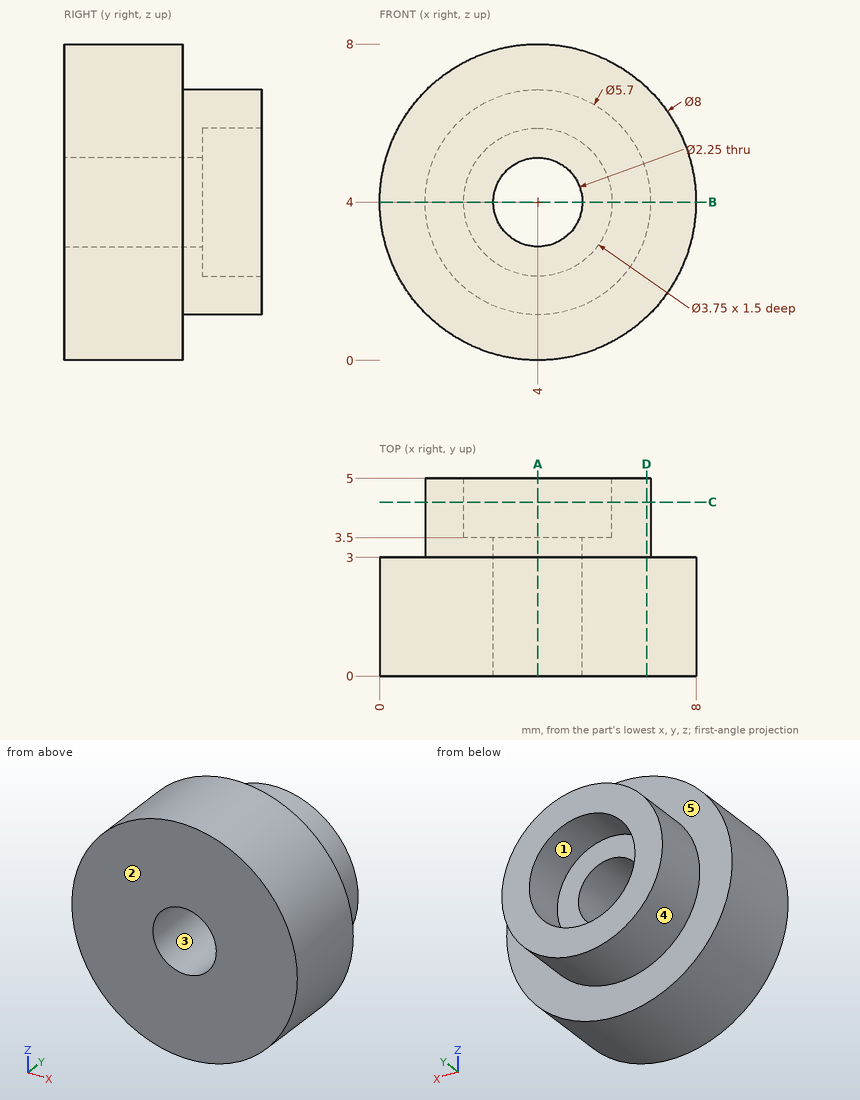
The drawing under review shows one solid part. Ordinate dimensions are in mm from its lowest x, y, z. A direction names the side the tool comes from. Round coordinates to 2 decimals unless told otherwise and drop trailing zeros. Loops run counter-clockwise (first coordinate to the right, second up) from the corner with the lowest first, then second, coordinate; pieces in that order, holes last. Notation, with made-up numbers: (23, 3) -> (66, 3) arc R29 cw to (66, 34) -> close; hole circle Ø10 at (-34, 34.25). An arc over 180 degrees is marked (long way). One line per question, with ' | ' between items. Start each with the question number.
Item 1: Add section C-C, the plane y = 4.4. Write out the cut boundary in (x, z) (3 decimals).
Item 2: Draft analysis for pull direction X (two halves, no side actions). For the marked faces 3, 4 and 5, state which applies: +X half, -X half, draft (parallel to the pull), parting line (faces both ways), or undercut.
Item 3: Add section B-B, the plane z = 4. Write out the cut boundary in (x, y) (3 decimals).
Item 4: For pin 1 (1.5 mm diameter, centred on y = 4, z = 5.5, fed in from -X); pin 2 (1.9 mm diameter, centred on x = 3.5, z = 3.5, fed in from +Y), all flat-tipped, find the tip position at first contact; note any pin that passes through.
Item 5: Add section D-D, the plane x = 6.75. Write out the cut boundary in (y, z).
Item 6: Wall thickness on line 1 along X through (y, z) = (4.1, 4) (3 decimals); line 2 along X through (y, z) = (1.15, 4) (3 decimals); line 3 along Y through (x, z) = (7, 2.5): over which ranges is each line inside the solid? List them lowest first. Write a range as [from, to].
Item 7: Machinability: for the marked faces 1 and 2, which of the approach directions +Z, -Z, +X, -X, +Y, -Y give a long, thin tool a straight path to every point of the face, cutting with its end or side? Answer none if there is none.
Item 8: Add section A-A, the plane x = 4. Write out the cut boundary in (y, z) (3 decimals), then the cut area to 3 significant figures.
Return value:
1) outline: circle Ø5.7 at (4, 4); hole circle Ø3.75 at (4, 4)
2) face 3: undercut | face 4: parting line | face 5: draft
3) outline: (0, 0) -> (2.875, 0) -> (2.875, 3.5) -> (2.125, 3.5) -> (2.125, 5) -> (1.15, 5) -> (1.15, 3) -> (0, 3) -> close; (5.125, 0) -> (8, 0) -> (8, 3) -> (6.85, 3) -> (6.85, 5) -> (5.875, 5) -> (5.875, 3.5) -> (5.125, 3.5) -> close
4) pin 1: stops at x = 1.25 | pin 2: stops at y = 3.5
5) outline: (0, 1.1) -> (3, 1.1) -> (3, 3.25) -> (5, 3.25) -> (5, 4.75) -> (3, 4.75) -> (3, 6.9) -> (0, 6.9) -> close
6) line 1: x = [1.15, 2.125], [5.875, 6.85] | line 2: x = [0, 2.875], [5.125, 8] | line 3: y = [0, 3]
7) face 1: +Y | face 2: +Z, -Z, +X, -X, -Y
8) outline: (0, 0) -> (3, 0) -> (3, 1.15) -> (5, 1.15) -> (5, 2.125) -> (3.5, 2.125) -> (3.5, 2.875) -> (0, 2.875) -> close; (0, 5.125) -> (3.5, 5.125) -> (3.5, 5.875) -> (5, 5.875) -> (5, 6.85) -> (3, 6.85) -> (3, 8) -> (0, 8) -> close | area: 21.9 mm2
